from build123d import *

# Parameters (mm, degrees)
ESQUISSE1_W              = 120
ESQUISSE1_H              = 60
BOSS_EXTRU_1_DEPTH       = 80
CHANFREIN1_SIZE          = 15
CHANFREIN2_SIZE          = 15
ENL_V_MAT_EXTRU_1_DEPTH  = 55
ESQUISSE3_R              = 4.5
ESQUISSE3_R_2            = 4.15
ESQUISSE3_R_3            = 9.675
ESQUISSE3_R_4            = 3.675
ENL_V_MAT_EXTRU_2_DEPTH  = 10
ESQUISSE4_R              = 5.1
ENL_V_MAT_EXTRU_3_DEPTH  = 10
ESQUISSE5_R              = 5.1
ENL_V_MAT_EXTRU_4_DEPTH  = 10
CHANFREIN3_SIZE          = 5
ESQUISSE7_W              = 15
ESQUISSE7_H              = 45
ENL_V_MAT_EXTRU_5_DEPTH  = 15
CHANFREIN5_SIZE          = 5
ESQUISSE8_W              = 25
ESQUISSE8_H              = 2
BOSS_EXTRU_2_DEPTH       = 6
ESQUISSE10_W             = 40
ESQUISSE10_H             = 10
BOSS_EXTRU_4_DEPTH       = 30
ESQUISSE11_W             = 40
ESQUISSE11_H             = 10
BOSS_EXTRU_5_DEPTH       = 30
ESQUISSE12_R             = 2.3
ENL_V_MAT_EXTRU_7_DEPTH  = 15
ESQUISSE13_R             = 2.3
ENL_V_MAT_EXTRU_8_DEPTH  = 16
ESQUISSE14_R             = 2.3
ENL_V_MAT_EXTRU_9_DEPTH  = 10
ESQUISSE15_R             = 3.2
ESQUISSE15_R_2           = 3.25
BOSS_EXTRU_6_DEPTH       = 3.4
ESQUISSE16_R             = 2.3
ENL_V_MAT_EXTRU_10_DEPTH = 5
ESQUISSE18_W             = 15
ESQUISSE18_H             = 12
ENL_V_MAT_EXTRU_13_DEPTH = 9
CONG_1_R                 = 5


with BuildPart() as part:
    # Esquisse1 → Boss.-Extru.1 (new body)
    with BuildSketch(Plane.XY):
        Rectangle(ESQUISSE1_W, ESQUISSE1_H)
    extrude(amount=-BOSS_EXTRU_1_DEPTH)

    # Chanfrein1
    chanfrein1_edges = [part.edges().sort_by_distance(p)[0] for p in [
        (60, 0, 0),
    ]]
    chamfer(chanfrein1_edges, length=CHANFREIN1_SIZE)

    # Chanfrein2
    chanfrein2_edges = [part.edges().sort_by_distance(p)[0] for p in [
        (-60, 0, 0),
    ]]
    chamfer(chanfrein2_edges, length=CHANFREIN2_SIZE)

    # Esquisse2 → Enlèv. mat.-Extru.1 (cut)
    with BuildSketch(Plane(origin=(0, 30, 0), x_dir=(1, 0, 0), z_dir=(0, 1, 0))):
        Polygon((-54, 15), (-54, 74), (54, 74), (54, 15), (45, 3), (-45, 3), align=None)
    extrude(amount=-ENL_V_MAT_EXTRU_1_DEPTH, mode=Mode.SUBTRACT)

    # Esquisse3 → Enlèv. mat.-Extru.2 (cut)
    with BuildSketch(Plane.XY):
        with Locations((0, 12)):
            Circle(ESQUISSE3_R)
        with Locations((-35, 18)):
            Circle(ESQUISSE3_R_2)
        with Locations((26.73, -5.87)):
            Circle(ESQUISSE3_R_3)
        with Locations((-26.73, -5.87)):
            Circle(ESQUISSE3_R_3)
        with Locations((39.34, 0)):
            Circle(ESQUISSE3_R_4)
        with Locations((-39.34, -12.37)):
            Circle(ESQUISSE3_R_4)
    extrude(amount=-ENL_V_MAT_EXTRU_2_DEPTH, mode=Mode.SUBTRACT)

    # Esquisse4 → Enlèv. mat.-Extru.3 (cut)
    with BuildSketch(Plane(origin=(22.5, 0, 22.5), x_dir=(0.7071067811865464, 0, -0.7071067811865488), z_dir=(0.7071067811865488, 0, 0.7071067811865464))):
        with Locations((42.819805153, 0)):
            Circle(ESQUISSE4_R)
    extrude(amount=-ENL_V_MAT_EXTRU_3_DEPTH, mode=Mode.SUBTRACT)

    # Esquisse5 → Enlèv. mat.-Extru.4 (cut)
    with BuildSketch(Plane(origin=(-22.5, 0, 22.5), x_dir=(0.7071067811865464, 0, 0.7071067811865488), z_dir=(-0.7071067811865488, 0, 0.7071067811865464))):
        with Locations((-42.819805153, 0)):
            Circle(ESQUISSE5_R)
    extrude(amount=-ENL_V_MAT_EXTRU_4_DEPTH, mode=Mode.SUBTRACT)

    # Chanfrein3
    chanfrein3_edges = [part.edges().sort_by_distance(p)[0] for p in [
        (52.5, -30, -7.5),
        (0, -30, 0),
        (-52.5, -30, -7.5),
        (60, -30, -47.5),
        (-60, -30, -47.5),
    ]]
    chamfer(chanfrein3_edges, length=CHANFREIN3_SIZE)

    # Esquisse7 → Enlèv. mat.-Extru.5 (cut)
    with BuildSketch(Plane(origin=(0, 0, -80), x_dir=(-1, 0, 0), z_dir=(0, 0, -1))):
        with Locations((0, -0.81)):
            Rectangle(ESQUISSE7_W, ESQUISSE7_H)
    extrude(amount=-ENL_V_MAT_EXTRU_5_DEPTH, mode=Mode.SUBTRACT)

    # Chanfrein5
    chanfrein5_edges = [part.edges().sort_by_distance(p)[0] for p in [
        (0, -30, -80),
    ]]
    chamfer(chanfrein5_edges, length=CHANFREIN5_SIZE)

    # Esquisse8 → Boss.-Extru.2 (add)
    with BuildSketch(Plane.XY):
        with Locations((0, 24)):
            Rectangle(ESQUISSE8_W, ESQUISSE8_H)
    extrude(amount=-BOSS_EXTRU_2_DEPTH)

    # Esquisse10 → Boss.-Extru.4 (add)
    with BuildSketch(Plane(origin=(60, 0, 0), x_dir=(0, 0, -1), z_dir=(1, 0, 0))):
        with Locations((45, -5)):
            Rectangle(ESQUISSE10_W, ESQUISSE10_H)
    extrude(amount=-BOSS_EXTRU_4_DEPTH)

    # Esquisse11 → Boss.-Extru.5 (add)
    with BuildSketch(Plane.ZY.offset(60)):
        with Locations((-45, -5)):
            Rectangle(ESQUISSE11_W, ESQUISSE11_H)
    extrude(amount=-BOSS_EXTRU_5_DEPTH)

    # Esquisse12 → Enlèv. mat.-Extru.7 (cut)
    with BuildSketch(Plane(origin=(0, 0, 0), x_dir=(1, 0, 0), z_dir=(0, 1, 0))):
        with Locations(Location((33.5, 55, 0), (0, 0, 270))):
            Circle(ESQUISSE12_R)
        with Locations(Location((48.5, 55, 0), (0, 0, 270))):
            Circle(ESQUISSE12_R)
        with Locations(Location((-33.5, 55, 0), (0, 0, 270))):
            Circle(ESQUISSE12_R)
        with Locations(Location((-48.5, 55, 0), (0, 0, 270))):
            Circle(ESQUISSE12_R)
    extrude(amount=-ENL_V_MAT_EXTRU_7_DEPTH, mode=Mode.SUBTRACT)

    # Esquisse13 → Enlèv. mat.-Extru.8 (cut)
    with BuildSketch(Plane(origin=(0, 30, 0), x_dir=(1, 0, 0), z_dir=(0, 1, 0))):
        with Locations(Location((-57, 65, 0), (0, 0, 270))):
            Circle(ESQUISSE13_R)
        with Locations(Location((-57, 35, 0), (0, 0, 270))):
            Circle(ESQUISSE13_R)
        with Locations(Location((57, 65, 0), (0, 0, 270))):
            Circle(ESQUISSE13_R)
        with Locations(Location((57, 35, 0), (0, 0, 270))):
            Circle(ESQUISSE13_R)
        with Locations(Location((0, 77, 0), (0, 0, 270))):
            Circle(ESQUISSE13_R)
    extrude(amount=-ENL_V_MAT_EXTRU_8_DEPTH, mode=Mode.SUBTRACT)

    # Esquisse14 → Enlèv. mat.-Extru.9 (cut)
    with BuildSketch(Plane(origin=(0, 0, -80), x_dir=(-1, 0, 0), z_dir=(0, 0, -1))):
        with Locations((19, 10)):
            Circle(ESQUISSE14_R)
        with Locations((19, -10)):
            Circle(ESQUISSE14_R)
        with Locations((-19, -10)):
            Circle(ESQUISSE14_R)
        with Locations((-19, 10)):
            Circle(ESQUISSE14_R)
    extrude(amount=-ENL_V_MAT_EXTRU_9_DEPTH, mode=Mode.SUBTRACT)

    # Esquisse15 → Boss.-Extru.6 (add)
    with BuildSketch(Plane(origin=(0, 0, -3), x_dir=(-1, 0, 0), z_dir=(0, 0, -1))):
        with Locations(Location((17, 11, 0), (0, 0, 180))):
            Circle(ESQUISSE15_R)
        with Locations(Location((-17, 11, 0), (0, 0, 180))):
            Circle(ESQUISSE15_R_2)
    extrude(amount=BOSS_EXTRU_6_DEPTH)

    # Esquisse16 → Enlèv. mat.-Extru.10 (cut)
    with BuildSketch(Plane(origin=(0, 0, -6.4), x_dir=(-1, 0, 0), z_dir=(0, 0, -1))):
        with Locations((17, 11)):
            Circle(ESQUISSE16_R)
        with Locations((-17, 11)):
            Circle(ESQUISSE16_R)
    extrude(amount=-ENL_V_MAT_EXTRU_10_DEPTH, mode=Mode.SUBTRACT)

    # Esquisse18 → Enlèv. mat.-Extru.13 (cut)
    with BuildSketch(Plane(origin=(0, -25, 0), x_dir=(1, 0, 0), z_dir=(0, 1, 0))):
        with Locations((0, 9)):
            Rectangle(ESQUISSE18_W, ESQUISSE18_H)
        with Locations((0, 36)):
            Rectangle(ESQUISSE18_W, ESQUISSE18_H)
    extrude(amount=-ENL_V_MAT_EXTRU_13_DEPTH, mode=Mode.SUBTRACT)

    # Congé1
    cong_1_edges = [part.edges().sort_by_distance(p)[0] for p in [
        (-60, 2.5, -80),
        (60, 2.5, -80),
    ]]
    fillet(cong_1_edges, radius=CONG_1_R)


solid = part.part
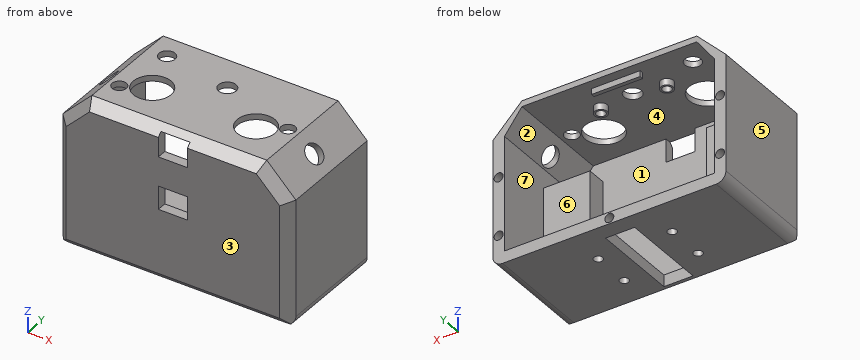
Verification items for the finished model (mm, model axes). Face numbers are marked on the shaded views. A direction names the side the tool comes from. Coordinates: 2 decimals unless noted, no trailing zeros. Loops run counter-clockwise (first coordinate to the right, second up) from the corner with the lowest first, then second, coordinate; pieces in that order, holes last. Notation, with made-up numbers: (30.25, 44.25) -> (87.25, 44.25) arc R18 cw to (87.25, 51.25) -> close; hole circle Ø2 at (-17.5, 89.25). An arc over 180 degrees is marked (long way). Answer as CSV lines item,"result".
1) Cross-section at D-D, the plane z = -71. Record the cut outline in (x, y).
Found:
outline,"(-60, -25) -> (-55, -30) -> (55, -30) -> (60, -25) -> (60, 30) -> (54, 30) -> (54, -25) -> (-54, -25) -> (-54, 30) -> (-60, 30) -> close"
2) Thickness scan on L1, parallel to X at y = -8, z = -55; L2, parallel to X at y = 25.5, z = -65; L3, parallel to Z at x = 27, y = 9. Record the ranges inside material, lowest first. Write a range as from..to.
Found:
L1,"x = -60..-50.8, -46.2..-35.8, -31.2..-30, 30..31.2, 35.8..46.2, 50.8..60"
L2,"x = -60..-59.3, -54.7..-54, 54..54.7, 59.3..60"
L3,"z = -80..-74, -3..0"
3) Depth check by flat-ended pin: pin 1 (1.4 mm diameter, centred on x = 56, z = -65.5, fed in from +Y); pin 2 (2 mm diameter, centred on y = 23.5, z = -4.5, fed in from +X); pin 3 (4 mm diameter, centred on x = 19, y = -10, fed in from -Z). Enter the tip coordinate at first touch or a pass-through.
Found:
pin 1,"stops at y = 14"
pin 2,"stops at x = 50.5"
pin 3,"stops at z = -3"
4) Release check for a two-part mould opening along Y. For the marked faces 4, 5, 6 and 7 record: +Y half, -Y half, draft (parallel to the pull), parting line (faces both ways), or undercut.
Found:
face 4,"undercut"
face 5,"draft"
face 6,"+Y half"
face 7,"undercut"
5) Tool access check on the marked faces 1, 2 and 3. Record the directions out of +Z, -Z, +X, -X, +Y, -Y that give a thin tool (end or side, any length) a straight path to the whole face; none if there is none.
Found:
face 1,"none"
face 2,"+Y"
face 3,"+Z, -Z, +X, -X, -Y"
6) Cross-section at A-A, the plane x = 39.34. Record the cut outline in (y, z) (3 decimals).
Found:
outline,"(-30, -75) -> (-25, -80) -> (30, -80) -> (30, -74) -> (-25, -74) -> (-25, -3) -> (-3.675, -3) -> (-3.675, 0) -> (-25, 0) -> (-30, -5) -> close; (-10, -65) -> (0, -65) -> (0, -25) -> (-10, -25) -> close; (3.675, -3) -> (30, -3) -> (30, 0) -> (3.675, 0) -> close"
7) Cross-section at B-B, the plane y = -14. Count the separate pieces of the cut face and the enclosed holes in it, then the cut area to 3 significant figures.
Found:
separate pieces,"4"
enclosed holes,"0"
area,"1,630 mm2"
